Source: CAD feature listing. Evaluate the final solid. Frame: model axes, mm. Give positions to 0.01 mm unless a question says otherwise; leave off trailing zeros. Order: outer loops, then holes, each group sorted by start corner. A loop starts at its lowest first (then second) coordinate and runs counter-clockwise, first axis right, second up. Notation, with made-up numbers: M 87,33.25 L 108,33.25 A23 ccw 108,49.25 Z; hole C 0.5,19 d2. An arc over 180 degrees is marked long. Answer in a Markdown table with one row per item. Add a question column.
(1) Section query B-B, the plane z = 0. Return loops of the section in (x, y).
(2) Section query A-A, the plane x = 0. Return loops of the section in (y, z).
(3) Material intervals for line 1 along Z through (x, y) = (0, 0.3); line 2 along X through (y, z) = (0.5, 11); line 3 along Z through (x, y) = (-10, 0.2), sorted ascending.
(4) Pin query (flat end, axial travel): P1, Ø10, axis at x = -4.5, z = 10.5, coming from the -Y side; P2, Ø24, axis at x = 0, z = 0, coming from the -Y side. Return the tip coordinate at first contact, or that it passes through.
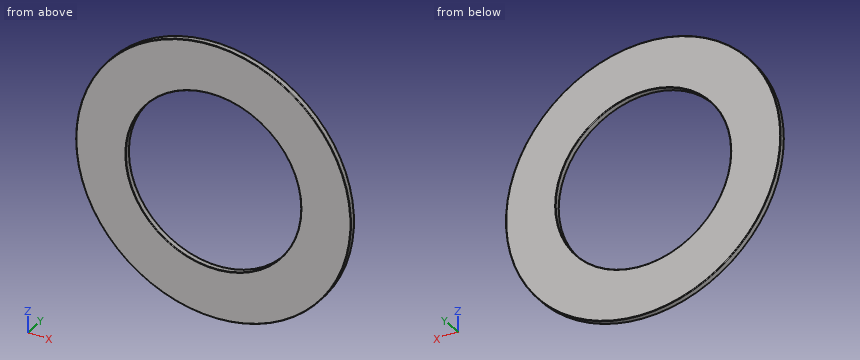
Autodesk Inventor part; units mm, degrees
ref_plane "YZ Plane" through (0, 0, 0) normal (1, 0, 0) x (0, 1, 0)
ref_plane "XZ Plane" through (0, 0, 0) normal (0, 1, 0) x (-1, 0, 0)
ref_plane "XY Plane" through (0, 0, 0) normal (0, 0, 1) x (1, 0, 0)
sketch "Skizze outline for Körper" plane through (0, 0, 0) normal (0, 0, 1) x (1, 0, 0)
  line L0 (-23.5, 0) -> (-15, 0)
  line L1 (-23.5, 1) -> (-23.5, 0)
  line L2 (-15, 1) -> (-23.5, 1)
  line L3 (-15, 0) -> (-15, 1)
revolve "Körper" add sketch "Skizze outline for Körper" angle 360 about axis through (0, -10, 0) along (0, 1, 0)
fillet "Rundung1" radius 0.1 4 edges at (23.5, 0, 0) (23.5, 1, 0) (15, 0, 0) (15, 1, 0)
sketch "Skizze" plane through (0, 0, 0) normal (0, 0, 1) x (1, 0, 0)
  line L0 (-23.5, 0) -> (-23.5, 1)
  line L1 (-23.5, 1) -> (-15, 1)
  line L2 (-15, 1) -> (-15, 0)
  line L3 (-94, 0) -> (-66, 0)
  line L4 (0, -0.5) -> (0, 3)
  dimension "d2" = 1
  dimension "d4" = 30
  dimension "d5" = 47
equation "\"d0\" = 0.1 * KB"
equation "\"d2\" = KB"
equation "\"d4\" = WD"
equation "\"d5\" = BD"
equation "\"WD\" = 30"
equation "\"BD\" = 47"
equation "\"KB\" = 1"
equation "\"BBA\" = 90deg"
equation "\"BR\" = 0.5 * BD"
equation "\"WR\" = 0.5 * WD"
properties part number "DIN 5405 T3 - AS3047 - 30 x 47 x 1" material "Stahl, weich"
Values follow:
| question | item | result |
|---|---|---|
| 1 | outline | M -23.5,0.1 A0.1 ccw -23.4,0 L -15.1,0 A0.1 ccw -15,0.1 L -15,0.9 A0.1 ccw -15.1,1 L -23.4,1 A0.1 ccw -23.5,0.9 Z; M 15,0.1 A0.1 ccw 15.1,0 L 23.4,0 A0.1 ccw 23.5,0.1 L 23.5,0.9 A0.1 ccw 23.4,1 L 15.1,1 A0.1 ccw 15,0.9 Z |
| 2 | outline | M 0,-23.4 A0.1 ccw 0.1,-23.5 L 0.9,-23.5 A0.1 ccw 1,-23.4 L 1,-15.1 A0.1 ccw 0.9,-15 L 0.1,-15 A0.1 ccw 0,-15.1 Z; M 0,15.1 A0.1 ccw 0.1,15 L 0.9,15 A0.1 ccw 1,15.1 L 1,23.4 A0.1 ccw 0.9,23.5 L 0.1,23.5 A0.1 ccw 0,23.4 Z |
| 3 | line 1 | z = -23.5 to -15, 15 to 23.5 |
| 3 | line 2 | x = -20.77 to -10.2, 10.2 to 20.77 |
| 3 | line 3 | z = -21.27 to -11.18, 11.18 to 21.27 |
| 4 | P1 | stops at y = 0 |
| 4 | P2 | passes through |
